The listing builds one solid part. Answer for the finished solid, in the listing's coordinates (mm). A direction names the side the tool comes from. Give positions to 0.01 mm unless a question says otherwise; leave off trailing zeros. Order: outer loops, then holes, each group sorted by start corner. A loop starts at its lowest first (then second) coordinate and runs counter-clockwise, first axis right, second up.
```python
from build123d import *

# Parameters (mm, degrees)
ESQUISSE1_W             = 126
ESQUISSE1_H             = 126
ESQUISSE1_W_2           = 116
ESQUISSE1_H_2           = 116
BOSS_EXTRU_1_DEPTH      = 25
ESQUISSE2_W             = 126
ESQUISSE2_H             = 126
BOSS_EXTRU_2_DEPTH      = 5
ENL_V_START             = -30
ESQUISSE3_W             = 28
ESQUISSE3_H             = 28
ESQUISSE3_W_2           = 33
ESQUISSE3_H_2           = 33
ENL_V_MAT_EXTRU_1_DEPTH = 30
BOSS_EXTRU_3_DEPTH      = 15
ESQUISSE5_W             = 15
ESQUISSE5_H             = 12
BOSS_EXTRU_4_DEPTH      = 5
CONG_1_R                = 5
D_GAGEMENT_M51_D        = 5.3
ESQUISSE9_W             = 10
ESQUISSE9_H             = 5
CONG_2_R                = 2


# Some blends are built 0.0001 mm under size
with BuildPart() as part:
    # Esquisse1 → Boss.-Extru.1 (new body)
    with BuildSketch(Plane.XY):
        Rectangle(ESQUISSE1_W, ESQUISSE1_H)
        Rectangle(ESQUISSE1_W_2, ESQUISSE1_H_2, mode=Mode.SUBTRACT)
    extrude(amount=BOSS_EXTRU_1_DEPTH)

    # Esquisse2 → Boss.-Extru.2 (add)
    with BuildSketch(Plane.XY.offset(25)):
        Rectangle(ESQUISSE2_W, ESQUISSE2_H)
    extrude(amount=BOSS_EXTRU_2_DEPTH)

    # Esquisse3 → Enlèv. mat.-Extru.1 (cut)
    with BuildSketch(Plane.XY.offset(30).offset(ENL_V_START)):
        with Locations((-49, 49)):
            Rectangle(ESQUISSE3_W, ESQUISSE3_H)
        with Locations((-46.5, -46.5)):
            Rectangle(ESQUISSE3_W_2, ESQUISSE3_H_2)
    extrude(amount=ENL_V_MAT_EXTRU_1_DEPTH, mode=Mode.SUBTRACT)

    # Esquisse4 → Boss.-Extru.3 (add)
    with BuildSketch(Plane(origin=(0, 0, 25), x_dir=(-1, 0, 0), z_dir=(0, 0, -1))):
        Polygon((35, 58), (35, 35), (58, 35), (58, 30), (30, 30), (30, 58), align=None)
        Polygon((58, -25), (25, -25), (25, -58), (30, -58), (30, -30), (58, -30), align=None)
    extrude(amount=BOSS_EXTRU_3_DEPTH)

    # Esquisse5 → Boss.-Extru.4 (add)
    with BuildSketch(Plane.XY):
        with Locations((-9.5, 69)):
            Rectangle(ESQUISSE5_W, ESQUISSE5_H)
        with Locations((45.5, 69)):
            Rectangle(ESQUISSE5_W, ESQUISSE5_H)
        with Locations((45.5, -69)):
            Rectangle(ESQUISSE5_W, ESQUISSE5_H)
        with Locations((-9.5, -69)):
            Rectangle(ESQUISSE5_W, ESQUISSE5_H)
    extrude(amount=BOSS_EXTRU_4_DEPTH)

    # Congé1
    cong_1_edges = [part.edges().sort_by_distance(p)[0] for p in [
        (-25, -41.5, 25),
        (16.5, -58, 25),
        (58, 0, 25),
        (14, 58, 25),
        (-30, 44, 25),
        (-44, 30, 25),
        (-58, 2.5, 25),
        (-41.5, -25, 25),
        (-63, 2.5, 30),
        (-49, 35, 30),
        (-35, 49, 30),
        (14, 63, 30),
        (63, 0, 30),
        (16.5, -63, 30),
        (-30, -46.5, 30),
        (-46.5, -30, 30),
        (58, -58, 12.5),
        (-25, -58, 17.5),
        (-25, -25, 17.5),
        (-58, -25, 17.5),
        (-58, 30, 17.5),
        (-30, 30, 17.5),
        (-30, 58, 17.5),
        (58, 58, 12.5),
        (53, -75, 2.5),
        (-2, -75, 2.5),
        (38, -75, 2.5),
        (-17, -75, 2.5),
        (-30, -63, 15),
        (-63, 35, 15),
        (-63, -30, 15),
        (-30, -30, 20),
        (-35, 35, 20),
        (53, 75, 2.5),
        (38, 75, 2.5),
        (-2, 75, 2.5),
        (-17, 75, 2.5),
        (63, 63, 15),
        (63, -63, 15),
        (-35, 63, 15),
    ]]
    fillet(cong_1_edges, radius=CONG_1_R - 0.0001)  # a hair under: the kernel refuses the full size

    # Dégagement M51 (through all)
    with Locations(Plane(origin=(0, 0, 0), x_dir=(1, 0, 0), z_dir=(0, 0, -1))):
        with Locations((-9.5, 69), (45.5, 69), (45.5, -69), (-9.5, -69)):
            Hole(D_GAGEMENT_M51_D / 2)

    # Esquisse9 → Enlèvement de matière-Révolution1 (revolve, cut)
    with BuildSketch(Plane.XY.offset(30)):
        with Locations((-53, 0)):
            Rectangle(ESQUISSE9_W, ESQUISSE9_H)
    revolve(axis=Axis((-63, 30, 30), (0, -1, 0)), mode=Mode.SUBTRACT)

    # Congé2
    # the kernel refuses this fillet: 2 mm, written as the material it takes off along each edge
    with BuildSketch(Plane(origin=(-48, -2.5, 30), x_dir=(1, 0, 0), z_dir=(0, 1, 0))) as cong_2_piece_1:
        with BuildLine():
            CenterArc((1.881943016, 2), CONG_2_R, 186.756327031, 83.243672969)
            ThreePointArc((-0.104167927, 1.764705882), (-0.026064627, 0.883888823), (0, 0))
            Line((0, 0), (1.881943016, 0))
        make_face()
    extrude(amount=5, mode=Mode.SUBTRACT)
    with BuildSketch(Plane(origin=(-43, 2.5, 30), x_dir=(0, 1, 0), z_dir=(-1, 0, 0))) as cong_2_piece_2_section:
        with BuildLine():
            CenterArc((CONG_2_R, CONG_2_R), CONG_2_R, 180, 90)
            Line((0, CONG_2_R), (0, 0))
            Line((0, 0), (CONG_2_R, 0))
        make_face()
    cong_2_piece_2 = extrude(amount=20, mode=Mode.PRIVATE)
    cong_2_piece_2 = cong_2_piece_2 & Plane(origin=(-63, 2.951907802, 30), x_dir=(1, 0, 0), z_dir=(0, 1, 0)) * Cylinder(15, 48, mode=Mode.PRIVATE)
    cong_2_piece_2 = cong_2_piece_2 - Plane(origin=(-63, 2.951907802, 30), x_dir=(1, 0, 0), z_dir=(0, -1, 0)) * Cylinder(5, 48, mode=Mode.PRIVATE)
    add(cong_2_piece_2, mode=Mode.SUBTRACT)
    with BuildSketch(Plane(origin=(-63, -2.5, 30), x_dir=(0, -1, 0), z_dir=(1, 0, 0))) as cong_2_piece_3_section:
        with BuildLine():
            CenterArc((CONG_2_R, CONG_2_R), CONG_2_R, 180, 90)
            Line((0, CONG_2_R), (0, 0))
            Line((0, 0), (CONG_2_R, 0))
        make_face()
    cong_2_piece_3 = extrude(amount=20, mode=Mode.PRIVATE)
    cong_2_piece_3 = cong_2_piece_3 & Plane(origin=(-63, -2.951907802, 30), x_dir=(1, 0, 0), z_dir=(0, 1, 0)) * Cylinder(15, 48, mode=Mode.PRIVATE)
    cong_2_piece_3 = cong_2_piece_3 - Plane(origin=(-63, -2.951907802, 30), x_dir=(1, 0, 0), z_dir=(0, -1, 0)) * Cylinder(5, 48, mode=Mode.PRIVATE)
    add(cong_2_piece_3, mode=Mode.SUBTRACT)
    with BuildSketch(Plane(origin=(-63, 2.5, 30), x_dir=(1, 0, 0), z_dir=(0, 0, -1))) as cong_2_piece_4_section:
        with BuildLine():
            CenterArc((CONG_2_R, -CONG_2_R), CONG_2_R, 90, 90)
            Line((0, -CONG_2_R), (0, 0))
            Line((0, 0), (CONG_2_R, 0))
        make_face()
    cong_2_piece_4 = extrude(amount=20, mode=Mode.PRIVATE)
    cong_2_piece_4 = cong_2_piece_4 & Plane(origin=(-63, 2.951908225, 30), x_dir=(1, 0, 0), z_dir=(0, 1, 0)) * Cylinder(15, 49, mode=Mode.PRIVATE)
    cong_2_piece_4 = cong_2_piece_4 - Plane(origin=(-63, 2.951908225, 30), x_dir=(1, 0, 0), z_dir=(0, -1, 0)) * Cylinder(5, 49, mode=Mode.PRIVATE)
    add(cong_2_piece_4, mode=Mode.SUBTRACT)
    with BuildSketch(Plane(origin=(-63, -2.5, 15), x_dir=(0, 0, -1), z_dir=(0, 1, 0))) as cong_2_piece_5:
        with BuildLine():
            CenterArc((1.881943016, -2), CONG_2_R, 90, 83.243672969)
            ThreePointArc((-0.104167927, -1.764705882), (-0.026064627, -0.883888823), (0, 0))
            Line((0, 0), (1.881943016, 0))
        make_face()
    extrude(amount=5, mode=Mode.SUBTRACT)
    with BuildSketch(Plane(origin=(-63, -2.5, 10), x_dir=(1, 0, 0), z_dir=(0, 0, 1))) as cong_2_piece_6_section:
        with BuildLine():
            CenterArc((CONG_2_R, -CONG_2_R), CONG_2_R, 90, 90)
            Line((0, -CONG_2_R), (0, 0))
            Line((0, 0), (CONG_2_R, 0))
        make_face()
    cong_2_piece_6 = extrude(amount=20, mode=Mode.PRIVATE)
    cong_2_piece_6 = cong_2_piece_6 - Plane(origin=(-63, -2.951908225, 30), x_dir=(1, 0, 0), z_dir=(0, -1, 0)) * Cylinder(5, 48, mode=Mode.PRIVATE)
    cong_2_piece_6 = cong_2_piece_6 & Plane(origin=(-63, -2.951908225, 30), x_dir=(1, 0, 0), z_dir=(0, 1, 0)) * Cylinder(15, 48, mode=Mode.PRIVATE)
    add(cong_2_piece_6, mode=Mode.SUBTRACT)
    with BuildSketch(Plane(origin=(-48, -7.20485754, 30), x_dir=(1, 0, 0), z_dir=(0, 1, 0))) as cong_2_piece_7a_section:
        with BuildLine():
            CenterArc((1.881943016, 2), CONG_2_R, 186.756327031, 83.243672969)
            ThreePointArc((-0.104167927, 1.764705882), (-0.026064627, 0.883888823), (0, 0))
            Line((0, 0), (1.881943016, 0))
        make_face()
    cong_2_piece_7a = extrude(amount=9.70485754, mode=Mode.PRIVATE)
    cong_2_piece_7a = split(cong_2_piece_7a, bisect_by=Plane(origin=(-47.580339744, -2.5, 29.603813963), z_dir=(0, -1, 0)), keep=Keep.TOP, mode=Mode.PRIVATE)
    with BuildSketch(Plane(origin=(-63, -2.5, 30), x_dir=(0, -1, 0), z_dir=(1, 0, 0))) as cong_2_piece_7b_section:
        with BuildLine():
            CenterArc((CONG_2_R, CONG_2_R), CONG_2_R, 180, 90)
            Line((0, CONG_2_R), (0, 0))
            Line((0, 0), (CONG_2_R, 0))
        make_face()
    cong_2_piece_7b = extrude(amount=20, mode=Mode.PRIVATE)
    cong_2_piece_7b = cong_2_piece_7b - Plane(origin=(-63, -2.951929409, 30), x_dir=(1, 0, 0), z_dir=(0, 1, 0)) * Cylinder(15, 48, mode=Mode.PRIVATE)
    cong_2_piece_7 = cong_2_piece_7a & cong_2_piece_7b
    add(cong_2_piece_7, mode=Mode.SUBTRACT)
    with BuildSketch(Plane(origin=(-43, 2.5, 30), x_dir=(0, 1, 0), z_dir=(-1, 0, 0))) as cong_2_piece_8a_section:
        with BuildLine():
            CenterArc((CONG_2_R, CONG_2_R), CONG_2_R, 180, 90)
            Line((0, CONG_2_R), (0, 0))
            Line((0, 0), (CONG_2_R, 0))
        make_face()
    cong_2_piece_8a = extrude(amount=20, mode=Mode.PRIVATE)
    cong_2_piece_8a = cong_2_piece_8a - Plane(origin=(-63, 2.951929409, 30), x_dir=(1, 0, 0), z_dir=(0, 1, 0)) * Cylinder(15, 48, mode=Mode.PRIVATE)
    with BuildSketch(Plane(origin=(-48, -2.5, 30), x_dir=(1, 0, 0), z_dir=(0, 1, 0))) as cong_2_piece_8b_section:
        with BuildLine():
            CenterArc((1.881943016, 2), CONG_2_R, 186.756327031, 83.243672969)
            ThreePointArc((-0.104167927, 1.764705882), (-0.026064627, 0.883888823), (0, 0))
            Line((0, 0), (1.881943016, 0))
        make_face()
    cong_2_piece_8b = extrude(amount=9.70485754, mode=Mode.PRIVATE)
    cong_2_piece_8b = split(cong_2_piece_8b, bisect_by=Plane(origin=(-47.580339744, 2.5, 29.603813963), z_dir=(0, 1, 0)), keep=Keep.TOP, mode=Mode.PRIVATE)
    cong_2_piece_8 = cong_2_piece_8a & cong_2_piece_8b
    add(cong_2_piece_8, mode=Mode.SUBTRACT)
    with BuildSketch(Plane(origin=(-63, 2.5, 30), x_dir=(1, 0, 0), z_dir=(0, 0, -1))) as cong_2_piece_9a_section:
        with BuildLine():
            CenterArc((CONG_2_R, -CONG_2_R), CONG_2_R, 90, 90)
            Line((0, -CONG_2_R), (0, 0))
            Line((0, 0), (CONG_2_R, 0))
        make_face()
    cong_2_piece_9a = extrude(amount=20, mode=Mode.PRIVATE)
    cong_2_piece_9a = cong_2_piece_9a - Plane(origin=(-63, 2.951929806, 30), x_dir=(1, 0, 0), z_dir=(0, 1, 0)) * Cylinder(15, 49, mode=Mode.PRIVATE)
    with BuildSketch(Plane(origin=(-63, -2.5, 15), x_dir=(0, 0, -1), z_dir=(0, 1, 0))) as cong_2_piece_9b_section:
        with BuildLine():
            CenterArc((1.881943016, -2), CONG_2_R, 90, 83.243672969)
            ThreePointArc((-0.104167927, -1.764705882), (-0.026064627, -0.883888823), (0, 0))
            Line((0, 0), (1.881943016, 0))
        make_face()
    cong_2_piece_9b = extrude(amount=9.70485754, mode=Mode.PRIVATE)
    cong_2_piece_9b = split(cong_2_piece_9b, bisect_by=Plane(origin=(-62.603813963, 2.5, 14.580339744), z_dir=(0, 1, 0)), keep=Keep.TOP, mode=Mode.PRIVATE)
    cong_2_piece_9 = cong_2_piece_9a & cong_2_piece_9b
    add(cong_2_piece_9, mode=Mode.SUBTRACT)
    with BuildSketch(Plane(origin=(-63, -2.5, 10), x_dir=(1, 0, 0), z_dir=(0, 0, 1))) as cong_2_piece_10a_section:
        with BuildLine():
            CenterArc((CONG_2_R, -CONG_2_R), CONG_2_R, 90, 90)
            Line((0, -CONG_2_R), (0, 0))
            Line((0, 0), (CONG_2_R, 0))
        make_face()
    cong_2_piece_10a = extrude(amount=20, mode=Mode.PRIVATE)
    cong_2_piece_10a = cong_2_piece_10a - Plane(origin=(-63, -2.951929806, 30), x_dir=(1, 0, 0), z_dir=(0, 1, 0)) * Cylinder(15, 48, mode=Mode.PRIVATE)
    with BuildSketch(Plane(origin=(-63, -7.20485754, 15), x_dir=(0, 0, -1), z_dir=(0, 1, 0))) as cong_2_piece_10b_section:
        with BuildLine():
            CenterArc((1.881943016, -2), CONG_2_R, 90, 83.243672969)
            ThreePointArc((-0.104167927, -1.764705882), (-0.026064627, -0.883888823), (0, 0))
            Line((0, 0), (1.881943016, 0))
        make_face()
    cong_2_piece_10b = extrude(amount=9.70485754, mode=Mode.PRIVATE)
    cong_2_piece_10b = split(cong_2_piece_10b, bisect_by=Plane(origin=(-62.603813963, -2.5, 14.580339744), z_dir=(0, -1, 0)), keep=Keep.TOP, mode=Mode.PRIVATE)
    cong_2_piece_10 = cong_2_piece_10a & cong_2_piece_10b
    add(cong_2_piece_10, mode=Mode.SUBTRACT)


solid = part.part
```
1) Find section A-A (x = 45.5). Write down the section's boundary in (y, z), then the cut area to 3 significant figures.
Geometry says:
outline: (-75, 0) - (-71.65, 0) - (-71.65, 5) - (-75, 5) - close; (-66.35, 0) - (-58, 0) - (-58, 20) arc R5 cw to (-53, 25) - (53, 25) arc R5 cw to (58, 20) - (58, 0) - (66.35, 0) - (66.35, 5) - (63, 5) - (63, 25) arc R5 ccw to (58, 30) - (-58, 30) arc R5 ccw to (-63, 25) - (-63, 5) - (-66.35, 5) - close; (71.65, 0) - (75, 0) - (75, 5) - (71.65, 5) - close
area: 947 mm2
2) For a pull along Y with two mould halves and no side action, classify faces 5 (the cylindrical face through (52, -73, 3)), 6 (the flat face through (-63, 2, 12)), 7 (the cylindrical face through (46.07, 71.59, 2.53)) as +Y half, -Y half, draft (parallel to the pull), parting line (faces both ways), or undercut.
Geometry says:
face 5: -Y half
face 6: draft
face 7: undercut
3) Straight lines are drawn through the part: probe 1 along Y at (x, z) = (-9.5, 2.7); probe 2 along X at (y, z) = (-69, 1.1); probe 3 along X at (y, z) = (-2, 1.5). For each, find the intervals that lie inside material, in ascending order.
Geometry says:
probe 1: y = -75 to -71.65, -66.35 to -58, 58 to 66.35, 71.65 to 75
probe 2: x = -17 to -12.15, -6.85 to -2, 38 to 42.85, 48.15 to 53
probe 3: x = -63 to -58, 58 to 63
4) A tool of negligible diameter and unlimited length cuts with its end or side. For faces 1 (the flat face through (-2, 66, 2)), 2 (the cylindrical face through (-49, 34, 28)), 3 (the flat face through (-30, -47, 18)), 4 (the flat face through (-30, 44, 15)), from which of +Z, -Z, +X, -X, +Y, -Y can it reach the whole face along a straight path? Write none if from no direction.
Geometry says:
face 1: +Z, -Z, +Y
face 2: +Z, -X, +Y
face 3: +Z, -Z, -X, -Y
face 4: -Z
5) Given P1, Ø2.5, axis at y = -67, z = 2, coming from the +X side; P2, Ø6, axis at x = -13, y = -68.5, coming from the +Z side; P3, Ø14, axis at x = -54, z = 21, coming from the +Y side, each flat-ended and moving along its own axis, determine where each tip first touches the part or whether it passes through.
Geometry says:
P1: stops at x = 53
P2: stops at z = 5
P3: stops at y = 35
6) Find section C-C (y = 61). Write down the section's boundary in (x, z).
Geometry says:
outline: (-34, 0) - (62, 0) - (62, 25) arc R4 ccw to (58, 29) - (-30, 29) arc R4 ccw to (-34, 25) - close
7) Find section B-B (x = 13.5). Write down the section's boundary in (y, z).
Geometry says:
outline: (-63, 0) - (-58, 0) - (-58, 20) arc R5 cw to (-53, 25) - (53, 25) arc R5 cw to (58, 20) - (58, 0) - (63, 0) - (63, 25) arc R5 ccw to (58, 30) - (-58, 30) arc R5 ccw to (-63, 25) - close
